Check sheet for the modelled part. Datum: model origin and axes. Units: mm. Face numbers are marked on the shaded views. A direction names the side the tool comes from. Round coordinates to 2 decimals unless told otherwise and drop trailing zeros. Loops run counter-clockwise (first coordinate to the right, second up) from the corner with the lowest first, then second, coordinate; pieces in that order, holes last. Notation, with made-up numbers: M -3,-15.75 L 32,-15.75 A15 cw 32,-5.75 Z; hole C 14.25,-4 d5. An arc over 180 degrees is marked long. Write item = value, one per line. Start each with the question number.
(1) Scan lines: L1, parallel to X at y = 2.55, z = -11.5; L2, parallel to X at y = 3.7, z = -5; L3, parallel to Z at x = 18, y = 3.05. Record each from-to range of solid material in increasing order. Write a range as from..to.
(2) Cross-section at A-A on z = -5. Record the boundary of the cut face in (x, y).
(3) Mould release check, pull along Z, two halves, no side actions. Record for the marked faces 5, 6 and 7: pulls with the +Z half, pulls with the -Z half, needs draft (parallel to the pull), parting line crosses it, or undercut.
(4) Cross-section at B-B on x = 15.25. Record the boundary of the cut face in (y, z), plus the area to 3 significant figures.
(5) Set-up check for the marked faces 1, 2, 3 and 4: record each of +Z, -Z, +X, -X, +Y, -Y from which the full face is reachable in a straight line by a thin tool's end or side.
(6) Go/stop test with flat-tipped pins: P1, Ø1.8, axis at y = 2.5, z = -5, coming from the +X side; P2, Ø2, axis at x = 4.5, y = 1, coming from the -Z side (3 decimals); P3, Ø4.5, axis at x = 4.5, z = -5, coming from the -Y side. Record where each tip stops, or that it passes through.
(7) Cross-section at C-C on z = -12.75. Record the boundary of the cut face in (x, y).
from build123d import *

# Parameters (mm, degrees)
SKETCH_1_R      = 2.4999999999999996
EXTRUDE_1_DEPTH = 4.5
EXTRUDE_START   = -1
SKETCH_3_R      = 2.4999999999999996
SKETCH_3_R_2    = 1.3499999999999994
EXTRUDE_3_DEPTH = 1
EXTRUDE_4_DEPTH = 15
FILLET_1_SIZE   = 3
FILLET_3_R      = 5
FILLET_4_R      = 8
FILLET_5_R      = 4
FILLET_6_R      = 3
FILLET_7_R      = 1
CHAMFER_3_SIZE  = 0.2
FILLET_8_R      = 2


# Some blends are built 0.0001 mm under size
with BuildPart() as part:
    # 草图1 → 凸台-拉伸1 (new body)
    with BuildSketch(Plane(origin=(0, 0, 0), x_dir=(1, 0, 0), z_dir=(0, 1, 0))):
        Polygon((6.500000000000001, 10), (9, 10), (9, 0), (0, 0), (0, 10), (2.499999999999998, 10), (2.500000000000002, 23), (6.500000000000003, 23), align=None)
        with Locations(Location((4.5, 5.000000000000001, 0), (0, 0, 270))):
            Circle(SKETCH_1_R, mode=Mode.SUBTRACT)
    extrude(amount=EXTRUDE_1_DEPTH)

    # 草图3 → 凸台-拉伸3 (add)
    with BuildSketch(Plane(origin=(0, 4.5, 0), x_dir=(1, 0, 0), z_dir=(0, 1, 0)).offset(EXTRUDE_START)):
        with Locations(Location((4.5, 5.000000000000001, 0), (0, 0, 270))):
            Circle(SKETCH_3_R)
        with Locations(Location((4.5, 5.000000000000001, 0), (0, 0, 270))):
            Circle(SKETCH_3_R_2, mode=Mode.SUBTRACT)
    extrude(amount=EXTRUDE_3_DEPTH)

    # 草图4 → 凸台-拉伸4 (add)
    with BuildSketch(Plane(origin=(6.499999999999999, 0, 8.7e-16), x_dir=(-2.9e-16, 0, -1), z_dir=(1, 0, -2.9e-16))):
        Polygon((23, 4.5), (19, 4.499999999999999), (19, 0), (23, 1.2e-16), align=None)
    extrude(amount=EXTRUDE_4_DEPTH)

    # 圆角1
    # a fillet whose section is not a circle: 3 mm, written as the material it takes off along each edge
    with BuildSketch(Plane(origin=(21.499999999999993, 12, -19.000000000000004), x_dir=(-1, 0, 0), z_dir=(0, -1, 0))) as fillet_1_piece_1:
        with BuildLine():
            Bezier((FILLET_1_SIZE, 0), (0, 0), (0, FILLET_1_SIZE), weights=[1, 0.818181818181818, 1])
            Line((0, FILLET_1_SIZE), (0, 0))
            Line((0, 0), (FILLET_1_SIZE, 0))
        make_face()
    extrude(amount=19.5, mode=Mode.SUBTRACT)

    # 圆角3
    fillet_3_edges = [part.edges().sort_by_distance(p)[0] for p in [
        (6.499999999999994, 2.2499999999999996, -19),
    ]]
    fillet(fillet_3_edges, radius=FILLET_3_R)

    # 圆角4
    fillet_4_edges = [part.edges().sort_by_distance(p)[0] for p in [
        (2.500000000000002, 2.25, -23),
    ]]
    fillet(fillet_4_edges, radius=FILLET_4_R)

    # 圆角5
    # the kernel refuses this fillet: 4 mm, written as the material it takes off along each edge
    with BuildSketch(Plane(origin=(9, -10, 0), x_dir=(-1, 0, 0), z_dir=(0, 1, 0))) as fillet_5_piece_1:
        with BuildLine():
            CenterArc((FILLET_5_R, -FILLET_5_R), FILLET_5_R, 90, 90)
            Line((0, -FILLET_5_R), (-FILLET_5_R * 0.02, -FILLET_5_R))
            Line((-FILLET_5_R * 0.02, -FILLET_5_R), (-FILLET_5_R * 0.02, FILLET_5_R * 0.02))
            Line((-FILLET_5_R * 0.02, FILLET_5_R * 0.02), (FILLET_5_R, FILLET_5_R * 0.02))
            Line((FILLET_5_R, FILLET_5_R * 0.02), (FILLET_5_R, 0))
        make_face()
    extrude(amount=24.5, mode=Mode.SUBTRACT)
    with BuildSketch(Plane(origin=(0, -10, 0), x_dir=(0, 0, -1), z_dir=(0, 1, 0))) as fillet_5_piece_2:
        with BuildLine():
            CenterArc((FILLET_5_R, -FILLET_5_R), FILLET_5_R, 90, 90)
            Line((-4.4e-16, -FILLET_5_R), (-FILLET_5_R * 0.02, -FILLET_5_R))
            Line((-FILLET_5_R * 0.02, -FILLET_5_R), (-FILLET_5_R * 0.02, FILLET_5_R * 0.02))
            Line((-FILLET_5_R * 0.02, FILLET_5_R * 0.02), (FILLET_5_R, FILLET_5_R * 0.02))
            Line((FILLET_5_R, FILLET_5_R * 0.02), (FILLET_5_R, 0))
        make_face()
    extrude(amount=24.5, mode=Mode.SUBTRACT)
    with BuildSketch(Plane(origin=(9, -9.27024810886958, -10), x_dir=(0, 0, 1), z_dir=(0, 1, 0))) as fillet_5_piece_3:
        with BuildLine():
            CenterArc((3.7080992435478315, -4), FILLET_5_R, 90, 67.97568716295783)
            Line((0, -2.499999999999999), (-0.07416198487095649, -2.469999999999999))
            ThreePointArc((-0.07416198487095649, -2.469999999999999), (-0.08000000000000007, -1.25), (-0.08000000000000007, 0))
            Line((-0.08000000000000007, 0), (0, 0.08000000000000007))
            Line((0, 0.08000000000000007), (3.7080992435478315, 0.08000000000000007))
            Line((3.7080992435478315, 0.08000000000000007), (3.7080992435478315, 0))
        make_face()
    extrude(amount=23.04049621773916, mode=Mode.SUBTRACT)
    with BuildSketch(Plane(origin=(0, -9.270248108869577, -10), x_dir=(1, 0, 0), z_dir=(0, 1, 0))) as fillet_5_piece_4:
        with BuildLine():
            CenterArc((4, -3.7080992435478306), FILLET_5_R, 112.0243128370422, 67.9756871629578)
            Line((0, -3.7080992435478306), (-0.08, -3.7080992435478306))
            Line((-0.08, -3.7080992435478306), (-0.08, 0))
            Line((-0.08, 0), (0, 0.08000000000000007))
            ThreePointArc((0, 0.08000000000000007), (1.249999999999999, 0.08000000000000007), (2.4699999999999975, 0.07416198487095649))
            Line((2.4699999999999975, 0.07416198487095649), (2.499999999999998, 0))
        make_face()
    extrude(amount=23.040496217739154, mode=Mode.SUBTRACT)

    # 圆角6
    fillet_6_edges = [part.edges().sort_by_distance(p)[0] for p in [
        (2.499999999999998, 2.25, -10),
        (6.500000000000001, 2.25, -10),
    ]]
    fillet(fillet_6_edges, radius=FILLET_6_R)

    # 圆角7
    fillet_7_edges = [part.edges().sort_by_distance(p)[0] for p in [
        (21.499999999999993, 2.25, -23.000000000000004),
    ]]
    fillet(fillet_7_edges, radius=FILLET_7_R - 0.0001)  # a hair under: the kernel refuses the full size

    # 倒角3
    chamfer_3_edges = [part.edges().sort_by_distance(p)[0] for p in [
        (4.5, 4.5, -6.3500000000000005),
        (15, 4.499999999999999, -19.000000000000004),
        (7.964466094067261, 4.5, -17.535533905932738),
        (7.964466094067261, 0, -17.535533905932738),
        (6.500000000000001, 4.5, -12.826901701916901),
        (6.500000000000001, 0, -12.826901701916901),
        (6.781019098475102, 4.5, -10.386072021741027),
        (6.781019098475102, 0, -10.386072021741027),
        (8.625307868699863, 0, -7.982209265909031),
        (8.625307868699863, 4.5, -7.982209265909031),
        (9, 4.5, -5.145950378226),
        (9, 0, -5.145950378226),
        (7.828427124746191, 4.5, -1.1715728752538102),
        (7.828427124746191, 0, -1.1715728752538102),
        (4.5, 0, 0),
        (4.5, 4.5, 0),
        (1.1715728752538102, 4.5, -1.1715728752538093),
        (1.1715728752538102, 0, -1.1715728752538093),
        (0, 0, -5.145950378226),
        (0, 4.5, -5.145950378226),
        (0.37469213130013657, 4.5, -7.982209265909032),
        (0.37469213130013657, 0, -7.982209265909032),
        (2.2189809015248967, 4.5, -10.386072021741029),
        (2.2189809015248967, 0, -10.386072021741029),
        (2.499999999999999, 0, -13.3269017019169),
        (2.499999999999999, 4.5, -13.3269017019169),
        (4.84314575050762, 4.5, -20.65685424949238),
        (4.84314575050762, 0, -20.65685424949238),
        (15.500049999999996, 4.5, -23.000000000000004),
        (15.500049999999996, 8e-17, -23.000000000000004),
        (21.207136070508422, 0, -22.70713607050843),
        (21.207136070508422, 4.5, -22.70713607050843),
        (20.675000000000082, 4.5, -19.82499999999992),
        (20.675000000000082, 0, -19.82499999999992),
        (4.500000000000001, 0, -7.5),
        (15, 0, -19.000000000000004),
    ]]
    chamfer(chamfer_3_edges, length=CHAMFER_3_SIZE)

    # 圆角8
    # the kernel refuses this fillet: 2 mm, written as the material it takes off along each edge
    with BuildSketch(Plane(origin=(4.5, 0.2, -5.000000000000001), x_dir=(-3.6e-16, 0, 1), z_dir=(-1, 0, -3.6e-16))) as fillet_8_piece_1:
        with BuildLine():
            CenterArc((4.499999999999999, 0.6717797887081369), FILLET_8_R, 180, 25.841932763167165)
            Line((2.499999999999999, 0.6717797887081369), (2.459999999999999, 0.6717797887081369))
            Line((2.459999999999999, 0.6717797887081369), (2.459999999999999, 0))
            Line((2.459999999999999, 0), (2.471715728752537, -0.02828427124746191))
            ThreePointArc((2.471715728752537, -0.02828427124746191), (2.5717157287525376, -0.1282842712474619), (2.6640000000000006, -0.21743559577416274))
            Line((2.6640000000000006, -0.21743559577416274), (2.7, -0.2))
        make_face()
    revolve(axis=Axis((4.5, 0.2, -5.000000000000001), (0, 1, 0)), mode=Mode.SUBTRACT)


solid = part.part
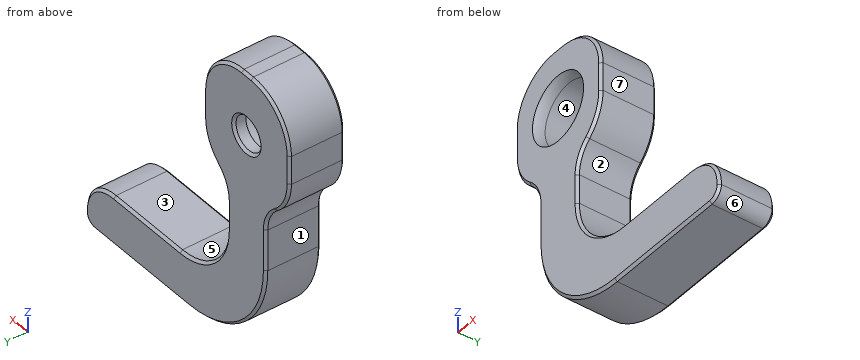
Result:
q1.L1 = 2.5..6.5
q1.L2 = 0..3.15, 5.85..9
q1.L3 = -23..-19
q2.outline = M 0,0.2 L 0.2,0 L 1.8,0 A2 ccw 2,0.87 L 2,3.5 L 3.15,3.5 L 3.15,4.3 L 2.95,4.5 L 0.2,4.5 L 0,4.3 Z; M 5.85,3.5 L 7,3.5 L 7,0.87 A2 ccw 7.2,0 L 8.8,0 L 9,0.2 L 9,4.3 L 8.8,4.5 L 6.05,4.5 L 5.85,4.3 Z
q3.face_5 = undercut
q3.face_6 = pulls with the -Z half
q3.face_7 = needs draft
q4.outline = M 0,-22.8 L 0.2,-23 L 4.3,-23 L 4.5,-22.8 L 4.5,-19.2 L 4.3,-19 L 0.2,-19 L 0,-19.2 Z
q4.area = 17.9 mm^2
q5.face_1 = -Z, -X, +Y, -Y
q5.face_2 = +X, +Y, -Y
q5.face_3 = +Z, +X, +Y, -Y
q5.face_4 = -Y
q6.P1 = 9
q6.P2 = -21.245
q6.P3 = 3.5
q7.outline = M 2.5,0.2 L 2.7,0 L 6.3,0 L 6.5,0.2 L 6.5,4.3 L 6.3,4.5 L 2.7,4.5 L 2.5,4.3 Z
